The listing builds one solid part. Answer for the finished solid, in the listing's coordinates (mm). Face numbers are marked on the shaded views. A direction names the side the tool comes from. Give positions to 0.01 mm unless a question says otherwise; leave off trailing zeros. Order: outer loops, then holes, each group sorted by start corner. A loop starts at its lowest first (then second) coordinate and runs counter-clockwise, first axis right, second up. Notation, with made-up numbers: M 65.5,8 L 83.5,8 A15 ccw 83.5,13 Z; hole C 82,78 d3. An arc over 180 degrees is marked long. Answer as a JSON object with one key per item and string values. Group by question number.
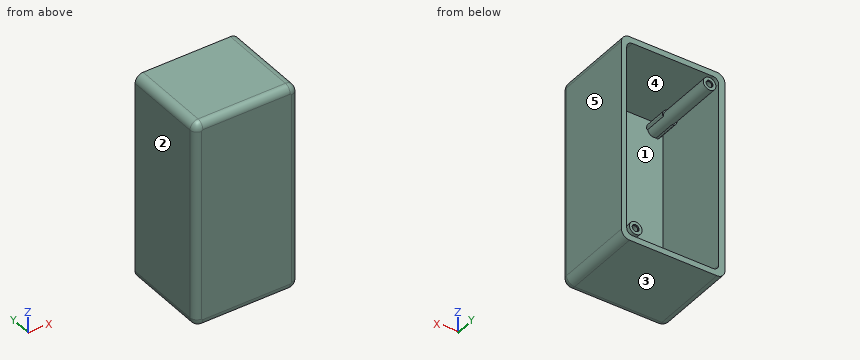
Autodesk Inventor part; units mm, degrees
ref_plane "YZ Plane" through (0, 0, 0) normal (1, 0, 0) x (0, 1, 0)
ref_plane "XZ Plane" through (0, 0, 0) normal (0, 1, 0) x (-1, 0, 0)
ref_plane "XY Plane" through (0, 0, 0) normal (0, 0, 1) x (1, 0, 0)
sketch "Sketch1" plane through (0, 0, 0) normal (0, 1, 0) x (-1, 0, 0)
  line L0 (-18.75, 52.5) -> (26.25, 52.5)
  line L1 (26.25, 52.5) -> (26.25, -37.5)
  line L2 (26.25, -37.5) -> (-18.75, -37.5)
  line L3 (-18.75, -37.5) -> (-18.75, 52.5)
  line L4 (26.25, 52.5) -> (-18.75, -37.5) construction
  line L5 (-16.4706, 50) -> (23.5294, 50)
  line L6 (23.5294, 50) -> (23.5294, -35)
  line L7 (23.5294, -35) -> (-16.4706, -35)
  line L8 (-16.4706, -35) -> (-16.4706, 50)
  line L9 (23.5294, 50) -> (-16.4706, -35) construction
  line L10 (23.5294, 50) -> (21.0294, 50)
  line L11 (21.0294, 50) -> (21.0294, 47.5)
  line L12 (21.0294, 47.5) -> (23.5294, 47.5)
  line L13 (23.5294, 47.5) -> (23.5294, 50)
  arc A0 (23.5294, 47.5) -> (21.0294, 50) centre (21.0294, 47.5) ccw
  line L14 (26.25, 52.5) -> (22.75, 52.5)
  line L15 (22.75, 52.5) -> (22.75, 49)
  line L16 (22.75, 49) -> (26.25, 49)
  line L17 (26.25, 49) -> (26.25, 52.5)
  line L18 (23.5294, -35) -> (21.0294, -35)
  line L19 (21.0294, -35) -> (21.0294, -32.5)
  line L20 (21.0294, -32.5) -> (23.5294, -32.5)
  line L21 (23.5294, -32.5) -> (23.5294, -35)
  line L22 (-16.4706, -35) -> (-13.9706, -35)
  line L23 (-13.9706, -35) -> (-13.9706, -32.5)
  line L24 (-13.9706, -32.5) -> (-16.4706, -32.5)
  line L25 (-16.4706, -32.5) -> (-16.4706, -35)
  line L26 (-16.4706, 50) -> (-13.9706, 50)
  line L27 (-13.9706, 50) -> (-13.9706, 47.5)
  line L28 (-13.9706, 47.5) -> (-16.4706, 47.5)
  line L29 (-16.4706, 47.5) -> (-16.4706, 50)
  arc A1 (-13.9706, 50) -> (-16.4706, 47.5) centre (-13.9706, 47.5) ccw
  arc A2 (-16.4706, -32.5) -> (-13.9706, -35) centre (-13.9706, -32.5) ccw
  arc A3 (21.0294, -35) -> (23.5294, -32.5) centre (21.0294, -32.5) ccw
  arc A4 (26.25, 49) -> (22.75, 52.5) centre (22.75, 49) ccw
  line L30 (26.25, -37.5) -> (22.75, -37.5)
  line L31 (22.75, -37.5) -> (22.75, -34)
  line L32 (22.75, -34) -> (26.25, -34)
  line L33 (26.25, -34) -> (26.25, -37.5)
  line L34 (-18.75, -37.5) -> (-15.25, -37.5)
  line L35 (-15.25, -37.5) -> (-15.25, -34)
  line L36 (-15.25, -34) -> (-18.75, -34)
  line L37 (-18.75, -34) -> (-18.75, -37.5)
  line L38 (-18.75, 52.5) -> (-15.25, 52.5)
  line L39 (-15.25, 52.5) -> (-15.25, 49)
  line L40 (-15.25, 49) -> (-18.75, 49)
  line L41 (-18.75, 49) -> (-18.75, 52.5)
  arc A5 (-15.25, 52.5) -> (-18.75, 49) centre (-15.25, 49) ccw
  arc A6 (-18.75, -34) -> (-15.25, -37.5) centre (-15.25, -34) ccw
  arc A7 (22.75, -37.5) -> (26.25, -34) centre (22.75, -34) ccw
  point P0 (0, 0)
  point P1 (26.25, 49)
  point P2 (22.75, 52.5)
  point P3 (-18.75, -34)
  point P4 (-16.4706, -32.5)
  point P5 (-15.9706, -34)
  point P6 (-16.4706, -34)
  point P7 (23.5294, -32.5)
  dimension "d0" = 45
  dimension "d1" = 90
  dimension "d2" = 40
  dimension "d3" = 85
  dimension "d8" = 2.5
  dimension "d9" = 2.5
extrude "Extrusion3" add sketch "Sketch1" along normal blind 2.5 contours L0 L15 L5 L39 | L39 L5 L8 L40 A5 | L40 L8 L36 L3 | A4 L16 L6 L5 L15 | L39 A1 L40 L8 L5 | L5 A1 L39 | L36 L8 L7 L35 A6 | L40 A1 L8 | L15 A0 L5 | L5 L6 L16 A0 L15 | L1 L32 L6 L16 | L5 L11 L12 L6 L20 L19 L7 L23 L24 L8 L28 L27 | L27 L28 A1 L40 L39 | L39 L40 A1 | L36 A2 L35 L7 L8 | L35 L7 L31 L2 | A0 L15 L16 L12 L11 | A0 L16 L15 | A7 L31 L7 L6 L32 | L6 A0 L16 | L24 L23 A2 L35 L36 | L36 L35 A2 | L35 A2 L7 | L32 A3 L6 | L6 L7 L31 A3 L32 | L7 A3 L31 | A3 L32 L31 L19 L20 | A3 L31 L32
extrude "Extrusion4" add sketch "Sketch1" along normal blind 37.5 contours L0 L15 L5 L39 | L39 L5 L8 L40 A5 | L40 L8 L36 L3 | A4 L16 L6 L5 L15 | L39 A1 L40 L8 L5 | L5 A1 L39 | L36 L8 L7 L35 A6 | L40 A1 L8 | L15 A0 L5 | L5 L6 L16 A0 L15 | L1 L32 L6 L16 | L36 A2 L35 L7 L8 | L8 A2 L36 | L35 L7 L31 L2 | A7 L31 L7 L6 L32 | L6 A0 L16 | L35 A2 L7 | L32 A3 L6 | L6 L7 L31 A3 L32 | L7 A3 L31
fillet "Fillet1" radius 3 8 edges at (-25.2249, 0, 51.4749) (-3.75, 0, 52.5) (17.7249, 0, 51.4749) (18.75, 0, 7.5) (17.7249, 0, -36.4749) (-3.75, 0, -37.5) (-25.2249, 0, -36.4749) (-26.25, 0, 7.5)
sketch "Sketch2" plane through (0, 2.5, 0) normal (0, 1, 0) x (1, 0, 0)
  arc A0 (16.4706, 32.5) -> (13.9706, 35) centre (13.9706, 32.5) ccw
  line L0 (13.9706, 35) -> (13.9706, 33.5)
  line L1 (16.4706, -47.5) -> (16.4706, 32.5)
  line L2 (16.4706, 32.5) -> (14.9706, 32.5)
  line L3 (14.9706, 32.5) -> (13.9706, 33.5)
  line L4 (14.4706, 33) -> (12.526, 31.0555)
  circle A1 centre (12.526, 31.0555) radius 2.75
  line L5 (-23.5294, 32.5) -> (-23.5294, -47.5)
  line L6 (-23.5294, -47.5) -> (-22.0294, -47.5)
  line L7 (-21.0294, -50) -> (13.9706, -50)
  line L8 (-21.0294, -50) -> (-21.0294, -48.5)
  line L9 (-21.0294, -48.5) -> (-22.0294, -47.5)
  line L10 (-21.5294, -48) -> (-19.5849, -46.0555)
  line L11 (-21.5294, -48) -> (-18.7794, -48) construction
  circle A2 centre (-19.5849, -46.0555) radius 2.75
  arc A3 (14.0518, 28.7675) -> (15.276, 31.0555) centre (12.526, 31.0555) ccw construction
  arc A4 (14.321, 28.3639) -> (15.7612, 31.0555) centre (12.526, 31.0555) ccw
  arc A5 (13.7826, 29.1712) -> (14.7909, 31.0555) centre (12.526, 31.0555) ccw
  arc A6 (13.7826, 29.1712) -> (14.321, 28.3639) centre (14.0518, 28.7675) ccw
  arc A7 (15.7612, 31.0555) -> (14.7909, 31.0555) centre (15.276, 31.0555) ccw
  arc A8 (10.7311, 33.747) -> (9.2909, 31.0555) centre (12.526, 31.0555) ccw
  arc A9 (9.2909, 31.0555) -> (10.2612, 31.0555) centre (9.776, 31.0555) ccw
  arc A10 (11.2694, 32.9398) -> (10.7311, 33.747) centre (11.0003, 33.3434) ccw
  arc A11 (11.2694, 32.9398) -> (10.2612, 31.0555) centre (12.526, 31.0555) ccw
  arc A12 (-17.79, -48.747) -> (-16.3497, -46.0555) centre (-19.5849, -46.0555) ccw
  arc A13 (-18.3283, -47.9398) -> (-17.32, -46.0555) centre (-19.5849, -46.0555) ccw
  arc A14 (-18.3283, -47.9398) -> (-17.79, -48.747) centre (-18.0591, -48.3434) ccw
  arc A15 (-16.3497, -46.0555) -> (-17.32, -46.0555) centre (-16.8349, -46.0555) ccw
  arc A16 (-21.3798, -43.3639) -> (-22.82, -46.0555) centre (-19.5849, -46.0555) ccw
  arc A17 (-22.82, -46.0555) -> (-21.8497, -46.0555) centre (-22.3349, -46.0555) ccw
  arc A18 (-20.8415, -44.1712) -> (-21.3798, -43.3639) centre (-21.1106, -43.7675) ccw
  arc A19 (-20.8415, -44.1712) -> (-21.8497, -46.0555) centre (-19.5849, -46.0555) ccw
  line L12 (-22.8137, -49.2843) -> (-20.2452, -46.7157) construction
  line L13 (-22.3894, -49.7085) -> (-19.8209, -47.14)
  line L14 (-20.6694, -46.2915) -> (-23.2379, -48.86)
  arc A20 (-23.2379, -48.86) -> (-22.3894, -49.7085) centre (-22.8137, -49.2843) ccw
  arc A21 (-19.8209, -47.14) -> (-20.6694, -46.2915) centre (-20.2452, -46.7157) ccw
  line L15 (12.9911, 31.5205) -> (15.9501, 34.4795) construction
  line L16 (13.4153, 31.0962) -> (16.3744, 34.0552)
  line L17 (15.5258, 34.9038) -> (12.5668, 31.9448)
  arc A22 (12.5668, 31.9448) -> (13.4153, 31.0962) centre (12.9911, 31.5205) ccw
  arc A23 (16.3744, 34.0552) -> (15.5258, 34.9038) centre (15.9501, 34.4795) ccw
  point P0 (0, 0)
  point P1 (14.848, 32.5289)
  point P2 (13.9995, 33.3774)
  point P3 (11.4261, 33.5759)
  point P4 (9.8188, 30.5722)
  point P5 (13.626, 28.535)
  point P6 (15.2333, 31.5387)
  point P7 (-21.9068, -47.5289)
  point P8 (-21.0583, -48.3774)
  point P9 (-18.4849, -48.5759)
  point P10 (-16.8777, -45.5722)
  point P11 (-20.6848, -43.535)
  point P12 (-22.2921, -46.5387)
  point P13 (15.2624, 34.6404)
  point P14 (16.111, 33.7918)
  dimension "d32" = 5.5
  dimension "d29" = 1.5
  dimension "d30" = 1.5
  dimension "d31" = 2.75
  dimension "d33" = 1.5
  dimension "d34" = 1.5
  dimension "d35" = 2.75
  dimension "d36" = 45
  dimension "d37" = 5.5
  dimension "d40" = 360
  dimension "d44" = 1.2
  dimension "d45" = 1.2
extrude "Extrusion5" add sketch "Sketch2" along normal blind 35 contours A0 L17 A23 L16 | A1 L16 A22 L4 | L4 A22 L17 A1 | A1 A7 A5 A6 A9 A11 A10 L17 A22 L16 | A1 A6 A5 A7 | A10 A11 A9 A1 | A2 L14 A21 L10 | L10 A21 L13 A2 | L13 A21 L14 A2 A17 A19 A18 A15 A13 A14 | A14 A13 A15 A2 | A2 A18 A19 A17
extrude "Extrusion6" add sketch "Sketch2" along normal blind 10 contours A7 A4 A6 A1 | A1 A9 A8 A10 | A2 L14 A21 L10 | L10 A21 L13 A2 | L13 A21 L14 A2 A17 A19 A18 A15 A13 A14 | A14 A13 A15 A2 | A2 A15 A12 A14 | A17 A16 A18 A2 | A2 A18 A19 A17
sketch "Sketch3" plane through (0, 37.5, 0) normal (0, 1, 0) x (1, 0, 0)
  arc A0 (-16.8349, -46.0555) -> (-16.8349, -46.0555) centre (-19.5849, -46.0555) ccw
  circle A1 centre (-19.5849, -46.0555) radius 1.5
  circle A2 centre (-19.5849, -46.0555) radius 1.25
  circle A3 centre (12.5766, 31.0622) radius 1.5
  circle A4 centre (12.5766, 31.0622) radius 1.25
  point P0 (0, 0)
  dimension "d50" = 3
  dimension "d51" = 2.5
  dimension "d52" = 3
  dimension "d53" = 2.5
extrude "Extrusion7" cut sketch "Sketch3" against normal blind 0.5 contours A1 | A3
extrude "Extrusion8" cut sketch "Sketch3" against normal blind 20 contours A2 | A4
extrude "Extrusion9" add sketch "Sketch2" along normal blind 32 contours L16 L3 L17 A0 | L16 A1 L3 | L3 A1 L17 | L13 A20 L14 L9 | L9 A2 L13 | L9 L14 A2
properties part number "proper shit spodnji"
Item 1: A tool of negligible diameter and unlimited length cuts with its end or side. For the marked faces 1 and 2, from which of +Z, -Z, +X, -X, +Y, -Y can it reach the whole face along a straight path? Write none if from no direction.
Item 2: Determine the mould class of the marked faces 3, 4 and 5 for opening direction Z: released by +Z, released by -Z, zero draft, split by the parting line, or undercut.
Item 3: Consider probe 1 along X at (y, z) = (30.5, -6); probe 2 along X at (y, z) = (18, 48); probe 3 along Z at (x, y) = (-16, 25). Determine where each line is inside the solid, lowest interval first. Write a range as from..to.
Item 4: Section A-A (x = 2) is taken. Determine the outline of the cut face in (y, z), and give its area (3 significant figures).
Item 5: Flat-ended cylindrical pins translate along their axes: P1, Ø8, axis at x = -16.5, z = 6, coming from the -Y side; P2, Ø1.8, axis at x = 12.58, z = -31.06, coming from the +Y side; P3, Ø5, axis at x = 6.5, z = 31, coming from the +Y side. Find the tip coordinate at first contact, or state that the pin passes through.
Item 6: Section C-C (z = 24) is taken. Determine the outline of the cut face in (x, y), and give its area (3 significant figures).
Item 7: Section B-B (y = 15) is taken. Determine the outline of the cut face in (x, z), and give its area (3 significant figures).
Item 8: Section D-D (y = 21) is taken. Determine the outline of the cut face in (x, z), and give its area (3 significant figures).
Values found:
{
 "1": {"face 1": "+Y", "face 2": "+Z, -Z, -X, +Y, -Y"},
 "2": {"face 3": "released by -Z", "face 4": "undercut", "face 5": "zero draft"},
 "3": {"probe 1": "x = -26.25..-23.53, 16.47..18.75", "probe 2": "x = -26.25..-23.48, -22.38..-17.64, 16.42..18.75", "probe 3": "z = -37.5..-35, 50..52.5"},
 "4": {"outline": "M 0,-34.5 A3 ccw 3,-37.5 L 37.5,-37.5 L 37.5,-35 L 2.5,-35 L 2.5,50 L 37.5,50 L 37.5,52.5 L 3,52.5 A3 ccw 0,49.5 Z", "area": "396 mm^2"},
 "5": {"P1": "stops at y = 0", "P2": "stops at y = 17.5", "P3": "stops at y = 2.5"},
 "6": {"outline": "M -26.25,3 A3 ccw -23.25,0 L 15.75,0 A3 ccw 18.75,3 L 18.75,37.5 L 16.47,37.5 L 16.47,2.5 L -23.53,2.5 L -23.53,37.5 L -26.25,37.5 Z", "area": "284 mm^2"},
 "7": {"outline": "M -26.25,-34 A3.5 ccw -22.75,-37.5 L 15.25,-37.5 A3.5 ccw 18.75,-34 L 18.75,49 A3.5 ccw 15.25,52.5 L -22.75,52.5 A3.5 ccw -26.25,49 Z; hole M -23.53,-32.5 A2.5 ccw -21.03,-35 L 13.97,-35 A2.5 ccw 15.26,-34.64 L 14,-33.38 A2.75 cw long 14.85,-32.53 L 16.11,-33.79 A2.5 ccw 16.47,-32.5 L 16.47,47.5 A2.5 ccw 13.97,50 L -21.03,50 A2.5 ccw -22.32,49.64 L -21.06,48.38 A2.75 cw long -21.91,47.53 L -23.17,48.79 A2.5 ccw -23.53,47.5 Z", "area": "697 mm^2"},
 "8": {"outline": "M -26.25,-34 A3.5 ccw -22.75,-37.5 L 15.25,-37.5 A3.5 ccw 18.75,-34 L 18.75,49 A3.5 ccw 15.25,52.5 L -22.75,52.5 A3.5 ccw -26.25,49 Z; hole M -23.53,-32.5 A2.5 ccw -21.03,-35 L 13.97,-35 A2.5 ccw 15.26,-34.64 L 14,-33.38 A2.75 cw long 14.85,-32.53 L 16.11,-33.79 A2.5 ccw 16.47,-32.5 L 16.47,47.5 A2.5 ccw 13.97,50 L -21.03,50 A2.5 ccw -22.32,49.64 L -21.06,48.38 A2.75 cw long -21.91,47.53 L -23.17,48.79 A2.5 ccw -23.53,47.5 Z; hole C -19.58,46.06 d2.5; hole C 12.58,-31.06 d2.5", "area": "687 mm^2"}
}
